The model under review builds one solid part; all positions refer to its coordinate system, in mm. A direction names the side the tool comes from. Round coordinates to 2 decimals unless told otherwise and drop trailing zeros. Loops run counter-clockwise (first coordinate to the right, second up) from the corner with the lowest first, then second, coordinate; pieces in that order, holes last. Notation, with made-up numbers: M -30,-1.75 L -11,-1.75 A27 cw -11,19.25 Z; hole C -31.75,23.25 d9. An arc over 180 degrees is marked long. One line per question, with ' | ' between items.
from build123d import *

# Parameters (mm, degrees)
SKETCH1_W           = 32
SKETCH1_H           = 28
BOSS_EXTRUDE1_DEPTH = 53
SKETCH2_W           = 26
SKETCH2_H           = 22
CUT_EXTRUDE1_DEPTH  = 56
SKETCH9_R           = 4.3
BOSS_EXTRUDE5_DEPTH = 53
SKETCH10_R          = 1.47
CUT_EXTRUDE5_DEPTH  = 53
SKETCH11_R          = 4.3
BOSS_EXTRUDE6_DEPTH = 53
SKETCH12_W          = 26
SKETCH12_H          = 3
BOSS_EXTRUDE7_DEPTH = 10
SKETCH13_R          = 1.47
CUT_EXTRUDE6_DEPTH  = 53
FILLET1_R           = 1


with BuildPart() as part:
    # Sketch1 → Boss-Extrude1 (new body)
    with BuildSketch(Plane(origin=(0, 0, 0), x_dir=(1, 0, 0), z_dir=(0, 1, 0))):
        with Locations((-16.792307692, 2.619230769)):
            Rectangle(SKETCH1_W, SKETCH1_H)
    extrude(amount=BOSS_EXTRUDE1_DEPTH)

    # Sketch2 → Cut-Extrude1 (cut)
    with BuildSketch(Plane(origin=(0, 53, 0), x_dir=(1, 0, 0), z_dir=(0, 1, 0))):
        with Locations((-16.792307692, 2.619230769)):
            Rectangle(SKETCH2_W, SKETCH2_H)
    extrude(amount=-CUT_EXTRUDE1_DEPTH, mode=Mode.SUBTRACT)

    # Sketch9 → Boss-Extrude5 (add)
    with BuildSketch(Plane(origin=(0, 53, 0), x_dir=(1, 0, 0), z_dir=(0, 1, 0))):
        with Locations((-32.792307692, -11.380769231)):
            Circle(SKETCH9_R)
    extrude(amount=-BOSS_EXTRUDE5_DEPTH)

    # Sketch10 → Cut-Extrude5 (cut)
    with BuildSketch(Plane(origin=(0, 53, 0), x_dir=(1, 0, 0), z_dir=(0, 1, 0))):
        with Locations((-32.792307692, -11.380769231)):
            Circle(SKETCH10_R)
    extrude(amount=-CUT_EXTRUDE5_DEPTH, mode=Mode.SUBTRACT)

    # Sketch11 → Boss-Extrude6 (add)
    with BuildSketch(Plane(origin=(0, 53, 0), x_dir=(1, 0, 0), z_dir=(0, 1, 0))):
        with Locations((-0.792307692, -11.380769231)):
            Circle(SKETCH11_R)
    extrude(amount=-BOSS_EXTRUDE6_DEPTH)

    # Sketch12 → Boss-Extrude7 (add)
    with BuildSketch(Plane.XY.offset(-13.619230769)):
        with Locations((-16.792307692, 1.5)):
            Rectangle(SKETCH12_W, SKETCH12_H)
    extrude(amount=BOSS_EXTRUDE7_DEPTH)

    # Sketch13 → Cut-Extrude6 (cut)
    with BuildSketch(Plane(origin=(0, 53, 0), x_dir=(1, 0, 0), z_dir=(0, 1, 0))):
        with Locations((-0.792307692, -11.380769231)):
            Circle(SKETCH13_R)
    extrude(amount=-CUT_EXTRUDE6_DEPTH, mode=Mode.SUBTRACT)

    # Fillet1
    fillet1_edges = [part.edges().sort_by_distance(p)[0] for p in [
        (-16.792307692, 53, -16.619230769),
        (-32.792307692, 53, -4.769230769),
        (-16.792307692, 0, -16.619230769),
        (-32.792307692, 0, -4.769230769),
        (-0.792307692, 0, -4.769230769),
        (-0.792307692, 53, -4.769230769),
        (-32.792307692, 26.5, -16.619230769),
        (-0.792307692, 26.5, -16.619230769),
    ]]
    fillet(fillet1_edges, radius=FILLET1_R)


solid = part.part
1) Add section C-C on y = 43. State the section outline as (x, z) points, then the cut area to 3 significant figures.
Output values:
outline: M -32.79,-15.62 A1 ccw -31.79,-16.62 L -1.79,-16.62 A1 ccw -0.79,-15.62 L -0.79,7.08 A4.3 ccw long -5.09,11.38 L -28.49,11.38 A4.3 ccw long -32.79,7.08 Z; hole C -32.79,11.38 d2.94; hole M -29.79,-13.62 L -3.79,-13.62 L -3.79,8.3 A4.3 cw -3.87,8.38 L -29.71,8.38 A4.3 cw -29.79,8.3 Z; hole C -0.79,11.38 d2.94 | area: 397 mm²
2) For line 1 (X direction, y = 41, z = 11.5); line 2 (Z direction, x = -18.5, y = 48.5); line 3 (X direction, y = 48, z = 12), list the stretches that pass through material, from the lowest coordinate up.
Output values:
line 1: x = -37.09 to -34.26, -31.33 to -28.49, -5.09 to -2.26, 0.67 to 3.51 | line 2: z = -16.62 to -13.62, 8.38 to 11.38 | line 3: x = -37.05 to -34.13, -31.46 to -28.54, -5.05 to -2.13, 0.54 to 3.46
3) Add section A-A on z = 5. State the section outline as (x, y) points, then the cut area to 3 significant figures.
Output values:
outline: M -32.79,1 A1 ccw -31.79,0 L -29.79,0 L -29.79,53 L -31.79,53 A1 ccw -32.79,52 Z; M -3.79,0 L -1.79,0 A1 ccw -0.79,1 L -0.79,52 A1 ccw -1.79,53 L -3.79,53 Z | area: 317 mm²
4) Machinability: for faces 4 (the flat face through (-32.792, 26, -4)), 5 (the flat face through (-17, 27, 8.381)), 6 (the flat face through (-17, 28, -13.619)), which of the approach directions +Z, -Z, +X, -X, +Y, -Y give a long, thin tool a straight path to every point of the face, cutting with its end or side? Answer none if there is none.
Output values:
face 4: -Z, -X, +Y, -Y | face 5: +Y, -Y | face 6: +Y
5) Add section D-D on z = -11. State the section outline as (x, y) points, then the cut area to 3 significant figures.
Output values:
outline: M -32.79,1 A1 ccw -31.79,0 L -1.79,0 A1 ccw -0.79,1 L -0.79,52 A1 ccw -1.79,53 L -3.79,53 L -3.79,3 L -29.79,3 L -29.79,53 L -31.79,53 A1 ccw -32.79,52 Z | area: 395 mm²
6) Add section B-B on x = -18.5. State the section outline as (y, z) points, then the cut area to 3 significant figures.
Output values:
outline: M 0,-15.62 A1 ccw 1,-16.62 L 52,-16.62 A1 ccw 53,-15.62 L 53,-13.62 L 3,-13.62 L 3,-3.62 L 0,-3.62 Z; M 0,8.38 L 53,8.38 L 53,11.38 L 0,11.38 Z | area: 348 mm²
7) Mouldability with a two-part tool opening along X and no side actions: class faces 1 (the flat face through (-0.792, 26, -4)), 2 (the flat face through (-17, 53, 10)), 3 (the flat face through (-17, 26, 11.381)) as +X half, -X half, draft (parallel to the pull), parting line (faces both ways), or undercut.
Output values:
face 1: +X half | face 2: draft | face 3: undercut
8) Insertion check: P1, Ø7, axis at y = 31, z = -0.5, coming from the -X side; P2, Ø8, axis at y = 17.5, z = -5, coming from the +X side; P3, Ø0.9, axis at x = -13, y = 2, coming from the +Z side; P4, Ø3.5, axis at x = -32.79, z = 11.38, coming from the -Y side. Each pin has a flat end and moves straight along its axis. Give the tip position at first contact, or say it passes through.
Output values:
P1: stops at x = -32.79 | P2: stops at x = -0.79 | P3: stops at z = 11.38 | P4: stops at y = 0
